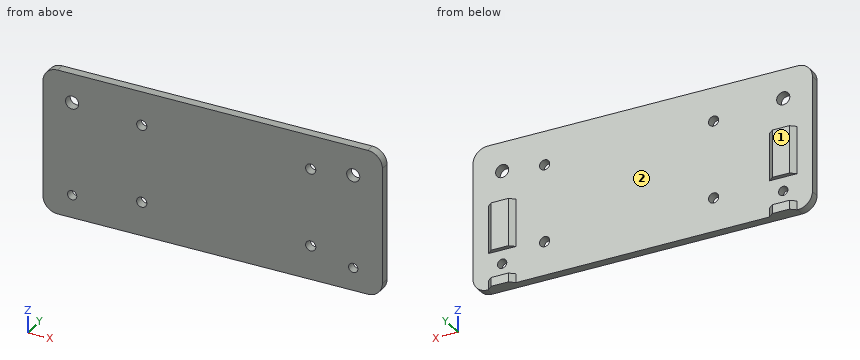
```python
from build123d import *

# Parameters (mm, degrees)
SKETCH_W        = 116.5
SKETCH_H        = 50
SKETCH_R        = 1.6
PAD_DEPTH       = 3
PAD001_DEPTH    = 50
PAD001_FACE18_R = 1.6
POCKET_DEPTH    = 255.213436
SKETCH002_W     = 9.5
SKETCH002_H     = 9.5
POCKET001_DEPTH = 1.5
SKETCH003_R     = 1.75
POCKET002_DEPTH = 5
POCKET003_DEPTH = 21
SKETCH004_R     = 1.6
PAD002_DEPTH    = 3
SKETCH005_R     = 2.25
POCKET004_DEPTH = 256.713436
FILLET_R        = 5


with BuildPart() as part:
    # Sketch → Pad (new body)
    with BuildSketch(Plane.XZ):
        Rectangle(SKETCH_W, SKETCH_H)
        with Locations((-48.25, 17.186)):
            Circle(SKETCH_R, mode=Mode.SUBTRACT)
        with Locations((-48.25, -17.186)):
            Circle(SKETCH_R, mode=Mode.SUBTRACT)
        with Locations((48.25, -17.186)):
            Circle(SKETCH_R, mode=Mode.SUBTRACT)
        with Locations((48.25, 17.186)):
            Circle(SKETCH_R, mode=Mode.SUBTRACT)
    extrude(amount=PAD_DEPTH)

    # Sketch001 (on Face1 of Pad) → Pad001 (join)
    with BuildSketch(Plane(origin=(0, 0, 25), x_dir=(-1, 0, 0), z_dir=(0, 0, 1))):
        Polygon((-51.2, -1.5), (-45.3, -1.5), (-43.5, 0), (-53, 0), align=None)
    pad001 = extrude(amount=-PAD001_DEPTH)

    # Pad001 Face18 → Pocket (cut, through all)
    with BuildSketch(Plane(origin=(48.25, 0, -17.186), x_dir=(-1, 0, 0), z_dir=(0, -1, 0))):
        Circle(PAD001_FACE18_R)
    pocket = extrude(amount=-POCKET_DEPTH, mode=Mode.SUBTRACT)

    # Sketch002 (on Face12 of Pocket) → Pocket001 (cut)
    with BuildSketch(Plane(origin=(0, 1.5, 0), x_dir=(1, 0, 0), z_dir=(0, 1, 0))):
        with Locations((48.25, 17.186)):
            Rectangle(SKETCH002_W, SKETCH002_H)
        with Locations((48.25, -17.186)):
            Rectangle(SKETCH002_W, SKETCH002_H)
    pocket001 = extrude(amount=-POCKET001_DEPTH, mode=Mode.SUBTRACT)

    # Mirrored: Pad001, Pocket, Pocket001 across YZ
    add(pad001.mirror(Plane.YZ))
    add(pocket.mirror(Plane.YZ), mode=Mode.SUBTRACT)
    add(pocket001.mirror(Plane.YZ), mode=Mode.SUBTRACT)

    # Sketch003 (on Face6 of Mirrored) → Pocket002 (cut)
    with BuildSketch(Plane(origin=(0, 0, 0), x_dir=(1, 0, 0), z_dir=(0, 1, 0))):
        with Locations((-24.35, -13.35)):
            Circle(SKETCH003_R)
        with Locations((33.65, -13.35)):
            Circle(SKETCH003_R)
        with Locations((33.65, 13.35)):
            Circle(SKETCH003_R)
        with Locations((-24.35, 13.35)):
            Circle(SKETCH003_R)
    extrude(amount=-POCKET002_DEPTH, mode=Mode.SUBTRACT)

    # Pocket002 Face5 → Pocket003 (cut)
    with BuildSketch(Plane(origin=(-48.25, 0.691558, 25), x_dir=(0, 1, 0), z_dir=(0, 0, 1))):
        Polygon((0.808442, -2.95), (0.808442, 2.95), (-0.691558, 4.75), (-0.691558, -4.75), align=None)
    pocket003 = extrude(amount=-POCKET003_DEPTH, mode=Mode.SUBTRACT)

    # Sketch004 (on Face11 of Pocket003) → Pad002 (join)
    with BuildSketch(Plane(origin=(0, 0, 0), x_dir=(1, 0, 0), z_dir=(0, 1, 0))):
        with Locations((-48.25, -17.186)):
            Circle(SKETCH004_R)
    pad002 = extrude(amount=-PAD002_DEPTH)

    # Sketch005 (on Face6 of Pad002) → Pocket004 (cut, through all)
    with BuildSketch(Plane(origin=(0, 0, 0), x_dir=(1, 0, 0), z_dir=(0, 1, 0))):
        with Locations((-48.25, -15)):
            Circle(SKETCH005_R)
    pocket004 = extrude(amount=-POCKET004_DEPTH, mode=Mode.SUBTRACT)

    # Mirrored001: Pocket003, Pad002, Pocket004 across YZ
    add(pocket003.mirror(Plane.YZ), mode=Mode.SUBTRACT)
    add(pad002.mirror(Plane.YZ))
    add(pocket004.mirror(Plane.YZ), mode=Mode.SUBTRACT)

    # Fillet
    fillet_edges = [part.edges().sort_by_distance(p)[0] for p in [
        (58.25, -1.5, 25),
        (58.25, -1.5, -25),
        (-58.25, -1.5, 25),
        (-58.25, -1.5, -25),
    ]]
    fillet(fillet_edges, radius=FILLET_R)


solid = part.part
```
Can you work these out from the model? Positions are in its coordinate system, mm. Face numbers are marked on the shaded views. Round coordinates to 2 decimals unless told otherwise and drop trailing zeros. Loops run counter-clockwise (first coordinate to the right, second up) from the corner with the lowest first, then second, coordinate; pieces in that order, holes last. Notation, with made-up numbers: M -33.75,61 L -10.75,61 A14 cw -10.75,82 Z; hole C 26.5,15 d8. An arc over 180 degrees is marked long. Answer in a Markdown table with one row per item.
1. Please list where these lines run through material, in increasing order: line 1 (Z direction, x = 33.65, y = -1.65); line 2 (X direction, y = -0.1, z = -13.5); line 3 (Z direction, x = -48.25, y = -1.9). Write a range as from..to.
Established:
| item | result |
|---|---|
| line 1 | -25..-15.1, -11.6..11.6, 15.1..25 |
| line 2 | -58.25..-26.09, -22.61..31.91, 35.39..58.25 |
| line 3 | -25..-18.79, -15.59..12.75, 17.25..25 |
2. I'm going to push flat-ended pins straight in: pin 1 Ø7 at (x, z) = (-48.25, 15) entering from +Y; pin 2 Ø1.9 at (x, z) = (48.25, -17.186) entering from +Y; pin 3 Ø0.8 at (x, y) = (-46.5, 0.5) entering from +Z. Where does each tip first touch, or does it pass through?
Established:
| item | result |
|---|---|
| pin 1 | y = 0 |
| pin 2 | through |
| pin 3 | z = 4 |
3. If we section it at D-D, the plane x = -48.25: Please give me the cut outline in (y, z), plus the area to 3 significant figures.
Established:
| item | result |
|---|---|
| outline | M -3,-25 L 1.5,-25 L 1.5,-21.94 L 0,-21.94 L 0,-18.79 L -3,-18.79 Z; M -3,-15.59 L 0,-15.59 L 0,-12.44 L 1.5,-12.44 L 1.5,4 L 0,4 L 0,12.75 L -3,12.75 Z; M -3,17.25 L 0,17.25 L 0,25 L -3,25 Z |
| area | 156 mm² |
4. If we section it at A-A, the plane x = -24.35: Please give me the cut outline in (y, z).
Established:
| item | result |
|---|---|
| outline | M -3,-25 L 0,-25 L 0,-15.1 L -3,-15.1 Z; M -3,-11.6 L 0,-11.6 L 0,11.6 L -3,11.6 Z; M -3,15.1 L 0,15.1 L 0,25 L -3,25 Z |
5. If we section it at B-B, the plane z = -7.5: Please give me the cut outline in (x, y).
Established:
| item | result |
|---|---|
| outline | M -58.25,-3 L 58.25,-3 L 58.25,0 L 53,0 L 51.2,1.5 L 45.3,1.5 L 43.5,0 L -43.5,0 L -45.3,1.5 L -51.2,1.5 L -53,0 L -58.25,0 Z |
6. Thinking about a two-plate mould opening in X: for the marked faces 1 and 2, which applies, pulls with the +X half, pulls with the -X half, needs draft (parallel to the pull), parting line crosses it, or undercut?
Established:
| item | result |
|---|---|
| face 1 | needs draft |
| face 2 | undercut |
7. If we section it at C-C, the plane y = -0.75: Give the number of separate pieces and of enclosed holes in the cut face, plus the area to 3 significant figures.
Established:
| item | result |
|---|---|
| separate pieces | 1 |
| enclosed holes | 8 |
| area | 5,720 mm² |
